The drawing under review shows one solid part. Ordinate dimensions are in mm from its lowest x, y, z. Coordinates: 2 decimals unless noted, no trailing zeros. Write each loop counter-clockwise with the first axis right and the second up, starting at its lowest first coordinate (ties: lowest second). Pieces come first, ordered by that corner, then holes.
1) Add section D-D, the plane z = 1.35. Give the number of separate pieces and of enclosed holes in the cut face, then the cut area to 3 significant figures.
2) Add section C-C, the plane y = 25. State the section outline as (x, z) points.
3) Add section A-A, the plane x = 14. State the section outline as (y, z) points.
4) Mouldability with a two-part tool opening along X and no side actions: class the marked faces 1, 2 and 3 as released by +X, released by -X, zero draft, split by the parting line, or undercut.
5) For line 1 (Y direction, x = 14, z = 1.7); line 2 (X direction, y = 7.25, z = 2.35) (1 decimal); line 3 (X direction, y = 14.5, z = 2.1) (1 decimal), list the stretches that pass through material, from the lowest coordinate up.
6) For P1, Ø1.5, axis at x = 3, z = 2, coming from the +Y side, flat-tipped, find the tip position at first contact; note if it passes through.
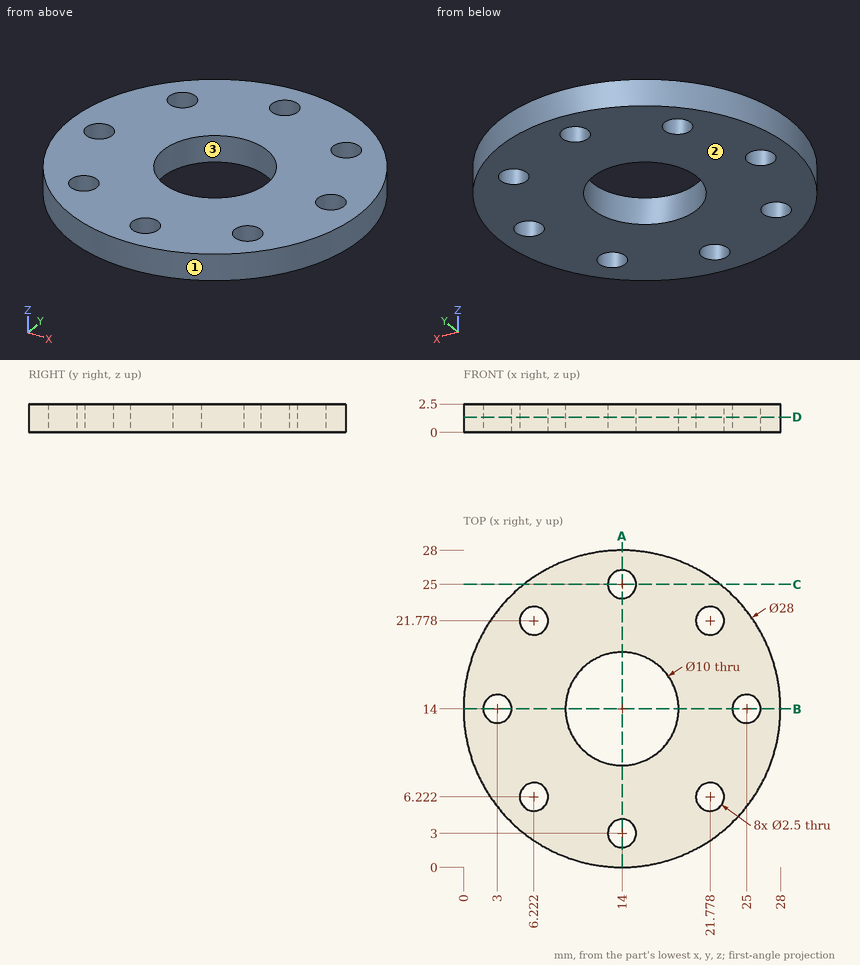
Geometry results:
1. separate pieces: 1
1. enclosed holes: 9
1. area: 498 mm2
2. outline: (5.34, 0) - (12.75, 0) - (12.75, 2.5) - (5.34, 2.5) - close; (15.25, 0) - (22.66, 0) - (22.66, 2.5) - (15.25, 2.5) - close
3. outline: (0, 0) - (1.75, 0) - (1.75, 2.5) - (0, 2.5) - close; (4.25, 0) - (9, 0) - (9, 2.5) - (4.25, 2.5) - close; (19, 0) - (23.75, 0) - (23.75, 2.5) - (19, 2.5) - close; (26.25, 0) - (28, 0) - (28, 2.5) - (26.25, 2.5) - close
4. face 1: split by the parting line
4. face 2: zero draft
4. face 3: undercut
5. line 1: y = 0 to 1.75, 4.25 to 9, 19 to 23.75, 26.25 to 28
5. line 2: x = 1.7 to 5.5, 6.9 to 21.1, 22.5 to 26.3
5. line 3: x = 0 to 1.9, 4.1 to 9, 19 to 23.9, 26.1 to 28
6. P1: stops at y = 23.54
